Design review of the part built by this model. Coordinates are the model's own, in mm. Face numbers are marked on the shaded views. A direction names the side the tool comes from. Round coordinates to 2 decimals unless told otherwise and drop trailing zeros. Loops run counter-clockwise (first coordinate to the right, second up) from the corner with the lowest first, then second, coordinate; pieces in that order, holes last. Notation, with made-up numbers: (36, 1) -> (40, 1) arc R12 ccw to (40, 23) -> close; hole circle Ø5 at (82, 18.5). An arc over 180 degrees is marked (long way). Answer as CSV lines item,"result". Start each with the question number.
```python
from build123d import *

# Parameters (mm, degrees)
F0_W     = 50.8
F0_H     = 50.8
F1_DEPTH = 88.9
F2_T     = -3.175
F3_W     = 3.175
F3_H     = 44.45
F4_DEPTH = 85.725
F5_W     = 44.45
F5_H     = 3.175
F6_DEPTH = 85.725


with BuildPart() as f1:
    # F0 (on Top) → F1 (new body)
    with BuildSketch(Plane.XY):
        Rectangle(F0_W, F0_H)
    extrude(amount=F1_DEPTH)

    # F2
    f2_openings = [f1.faces().sort_by_distance(p)[0] for p in [
        (0, 0, 88.9),
    ]]
    offset(amount=F2_T, openings=f2_openings)



with BuildPart() as f4:
    # F3 (on face) → F4 (new body)
    with BuildSketch(Plane.XY.offset(88.9)):
        with Locations((-0.0127, 0)):
            Rectangle(F3_W, F3_H)
    extrude(amount=-F4_DEPTH)


with BuildPart() as f1_1:
    add(f1.part)

    add(f4.part)  # F6 merges F4
    # F5 (on face) → F6 (join)
    with BuildSketch(Plane.XY.offset(3.175)):
        with Locations((0, -0.0127)):
            Rectangle(F5_W, F5_H)
    extrude(amount=F6_DEPTH)


solid = f1_1.part
```
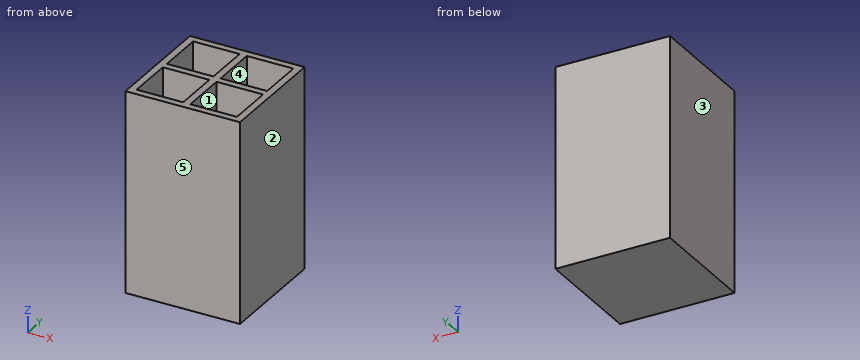
Q1. For pin 1 Ø10.5 at (x, y) = (12.5, 7) entering from +Z (3 decimals), flat-tipped, find the tip position at first contact; note if it passes through.
Q2. Add section A-A, the plane z = 55. Give the boundary of the cut face in (x, y) (3 decimals), and give its area (3 significant figures).
Q3. Machinability: for the marked faces 1 and 2, which of the approach directions +Z, -Z, +X, -X, +Y, -Y give a long, thin tool a straight path to every point of the face, cutting with its end or side? Answer none if there is none.
Q4. To check wall thickness, follow probe 1 along Y at (x, z) = (-15, 5) (3 decimals); probe 2 along Z at (x, y) = (20, 9.5) (3 decimals). State the ranges of each line that lie inside material, in increasing order. Write a range as from..to.
Q5. Mouldability with a two-part tool opening along Y and no side actions: class the marked faces 3, 4 and 5 as pulls with the +Y half, pulls with the -Y half, needs draft (parallel to the pull), parting line crosses it, or undercut.
Q6. Add section B-B, the plane x = 18. Give the boundary of the cut face in (y, z) (3 decimals), and give its area (3 significant figures).
Worked answers:
1,pin 1,"stops at z = 3.175"
2,outline,"(-25.4, -25.4) -> (25.4, -25.4) -> (25.4, 25.4) -> (-25.4, 25.4) -> close; hole (-22.225, -22.225) -> (-1.6, -22.225) -> (-1.6, -1.6) -> (-22.225, -1.6) -> close; hole (-22.225, 1.575) -> (-1.6, 1.575) -> (-1.6, 22.225) -> (-22.225, 22.225) -> close; hole (1.575, -22.225) -> (22.225, -22.225) -> (22.225, -1.6) -> (1.575, -1.6) -> close; hole (1.575, 1.575) -> (22.225, 1.575) -> (22.225, 22.225) -> (1.575, 22.225) -> close"
2,area,"877 mm^2"
3,face 1,"+Z"
3,face 2,"+Z, -Z, +X, +Y, -Y"
4,probe 1,"y = -25.4..-22.225, -1.6..1.575, 22.225..25.4"
4,probe 2,"z = 0..3.175"
5,face 3,"needs draft"
5,face 4,"undercut"
5,face 5,"pulls with the -Y half"
6,outline,"(-25.4, 0) -> (25.4, 0) -> (25.4, 88.9) -> (22.225, 88.9) -> (22.225, 3.175) -> (1.575, 3.175) -> (1.575, 88.9) -> (-1.6, 88.9) -> (-1.6, 3.175) -> (-22.225, 3.175) -> (-22.225, 88.9) -> (-25.4, 88.9) -> close"
6,area,"978 mm^2"
